Autodesk Inventor part; units mm, degrees
ref_plane "YZ Plane" through (0, 0, 0) normal (1, 0, 0) x (0, 1, 0)
ref_plane "XZ Plane" through (0, 0, 0) normal (0, 1, 0) x (-1, 0, 0)
ref_plane "XY Plane" through (0, 0, 0) normal (0, 0, 1) x (1, 0, 0)
sketch "Szkic1" plane through (0, 0, 0) normal (0, 0, 1) x (1, 0, 0)
  line L0 (0, 0) -> (-30, 30)
  line L1 (-30, 30) -> (-30, 27.1716)
  line L2 (-30, 27.1716) -> (-2.8284, 0)
  line L3 (-2.8284, 0) -> (0, 0)
  line L4 (-30, 27.1716) -> (-30.8284, 28)
  line L5 (-30.8284, 28) -> (-30.8284, 30)
  line L6 (-30.8284, 30) -> (-30, 30)
  dimension "d0" = 2
  dimension "d1" = 30
  dimension "d2" = 45
  dimension "d3" = 2
extrude "Wyciągnięcie proste1" add sketch "Szkic1" along normal blind 180.257
sketch "Szkic2" plane through (-30.8284, 28, 0) normal (-1, 0, 0) x (0, 0, 1)
  line L0 (0, 0) -> (0, -28)
  line L1 (0, 2) -> (180.257, 2)
  line L2 (0, -28) -> (0, 2)
  line L3 (0, 2) -> (30, 2)
  line L4 (0, 0) -> (180.257, 0)
  line L5 (30, 2) -> (0, -28)
  line L6 (180.257, 2) -> (180.257, -20)
  line L7 (180.257, 0) -> (180.257, -28)
  line L8 (180.257, 2) -> (142.1519, 2)
  line L9 (180.257, -20) -> (142.1519, 2)
  dimension "d6" = 45
  dimension "d7" = 30
  dimension "d8" = 22
extrude "Wyciągnięcie proste2" cut sketch "Szkic2" against normal through all contours L4 L5 L0 | L2 L1 L5 L4 | L9 L1 L6 L4 | L4 L6 L9
sketch "Szkic3" plane through (0, 0, 0) normal (0.7071, 0.7071, 0) x (-0.7071, 0.7071, 0)
  line L0 (42.4264, 30) -> (42.4264, 142.1519) construction
  line L1 (42.4264, 115.152) -> (23.012, 115.152) construction
  circle A0 centre (32.012, 135.152) radius 1.6
  circle A1 centre (23.012, 115.152) radius 1.6
  circle A2 centre (32.012, 33.9815) radius 1.6
  line L2 (41.598, 28) -> (41.598, 145.616)
  point P0 (0, 0)
  dimension "d17" = 3.2
  dimension "d37" = 9.586
  dimension "d38" = 5.9815
  dimension "d39" = 10.464
  dimension "d40" = 30.464
  dimension "d41" = 18.586
extrude "Wyciągnięcie proste3" cut sketch "Szkic3" against normal through all
chamfer "Faza1" distance 1.85 distance2 1.75 1 edges at (-15.1406, 15.1406, 115.152) measured on face at (-5.0469, 5.0469, 98.4697)
chamfer "Faza2" distance 1.85 distance2 1.75 1 edges at (-21.5045, 21.5045, 135.152) measured on face at (-4.6108, 4.6108, 98.4697)
chamfer "Faza3" distance 1.85 distance2 1.75 1 edges at (-21.5045, 21.5045, 33.9815) measured on face at (-4.6108, 4.6108, 98.4697)
sketch "Szkic4" plane through (-30.8284, 28, 28) normal (-1, 0, 0) x (0, 0, 1)
  circle A0 centre (34.7574, -13) radius 19.25
  line L0 (-28, -28) -> (152.257, -28)
  dimension "d29" = 62.7574
  dimension "d30" = 38.5
  dimension "d31" = 15
extrude "Wyciągnięcie proste4" cut sketch "Szkic4" against normal blind 22.5
sketch "Szkic5" plane through (0, 0, 0) normal (0.7071, 0.7071, 0) x (-0.7071, 0.7071, 0)
  line L0 (9.7782, 79.4999) -> (9.7782, 46.0149)
  line L1 (9.7782, 79.4999) -> (9.7782, 46.0149)
  ellipse E0 centre (16.4957, 62.7574) end of major axis (16.4957, 43.5074) minor radius 13.6118 (9.7782, 46.0149) -> (11.7782, 44.7005) ccw
  ellipse E1 centre (16.4957, 62.7574) end of major axis (16.4957, 43.5074) minor radius 13.6118 (11.7782, 80.8143) -> (9.7782, 79.4999) ccw
  ellipse E2 centre (23.2132, 62.7574) end of major axis (50.4368, 62.7574) minor radius 19.25 (41.598, 76.9547) -> (9.7782, 79.4999) ccw
  ellipse E3 centre (32.4056, 62.7574) end of major axis (32.4056, 43.5074) minor radius 13.6118 (43.0122, 74.8223) -> (41.598, 76.9547) ccw
  ellipse E4 centre (32.4056, 62.7574) end of major axis (32.4056, 43.5074) minor radius 13.6118 (41.598, 48.5601) -> (43.0122, 50.6925) ccw
  line L2 (43.0122, 74.8223) -> (43.0122, 50.6925)
  ellipse E5 centre (23.2132, 62.7574) end of major axis (50.4368, 62.7574) minor radius 19.25 (9.7782, 46.0149) -> (41.598, 48.5601) ccw
  ellipse E6 centre (21.2132, 62.7574) end of major axis (48.4368, 62.7574) minor radius 19.25 (11.7782, 44.7005) -> (42.4264, 50.6925) ccw
  ellipse E7 centre (21.2132, 62.7574) end of major axis (48.4368, 62.7574) minor radius 19.25 (42.4264, 74.8223) -> (11.7782, 80.8143) ccw
  line L3 (42.4264, 30) -> (42.4264, 50.6925)
  line L4 (42.4264, 74.8223) -> (42.4264, 50.6925)
  point P0 (0, 0)
  point P1 (41.598, 48.5601)
extrude "Wyciągnięcie proste5" cut sketch "Szkic5" against normal through all
properties part number "Bok2mm"
Here's how the part is built. I have some questions about the finished solid (model axes, mm). Round coordinates to 2 decimals unless told otherwise and drop trailing zeros. Loops run counter-clockwise (first coordinate to the right, second up) from the corner with the lowest first, then second, coordinate; pieces in that order, holes last. Notation, with made-up numbers: (23, -21.75) -> (32, -21.75) arc R7 ccw to (32, -15.75) -> close; hole circle Ø8 at (-14, -28). An arc over 180 degrees is marked (long way). Write each question's results on one line, items separated by ' | '.
(1) If I drill on L1, parallel to X at y = 2.5, z = 98.5; L2, parallel to X at y = 11, z = 87; L3, parallel to Y at x = -6.5, z = 128.5, over which ranges is the centre line in solid material (lowest first)?
Worked answers:
L1: -5.33 to -2.5 | L2: -13.83 to -11 | L3: 3.67 to 6.5
(2) We'd pull the mould along Z, two halves only. Please class faces 1 (the face through (-19.467, 18.134, 162.705)), 2 (the face through (-13.91, 11.08, 88.87)), 3 (the face through (-23.5, 21.2, 32.3)): released by +Z, released by -Z, zero draft, split by the parting line, or undercut.
Worked answers:
face 1: released by +Z | face 2: zero draft | face 3: undercut
(3) If we section it at B-B, the plane z = 17: List the corners of the cut face in (x, y) for me.
Worked answers:
outline: (-19.83, 17) -> (-2.83, 0) -> (0, 0) -> (-17, 17) -> close
(4) If we section it at A-A, the plane z = 107.5: List the corners of the cut face in (x, y) for me, then the cut area to 3 significant figures.
Worked answers:
outline: (-30.83, 28) -> (-2.83, 0) -> (0, 0) -> (-30, 30) -> (-30.83, 30) -> close | area: 82.9 mm2
(5) If we section it at C-C, the plane z = 166: List the corners of the cut face in (x, y) for me.
Worked answers:
outline: (-19.06, 16.23) -> (-2.83, 0) -> (0, 0) -> (-16.23, 16.23) -> close
(6) For P1, Ø8, axis at x = -15.5, y = 3, coming from the +Z side; P2, Ø10, axis at y = 23.5, z = 90, coming from the +X side; P3, Ø3, axis at y = 15, z = 110, coming from the +X side; P4, Ø4, axis at x = -15.5, z = 117.5, coming from the +Y side, each with a flat end and sliding along its axis, tell me the tip position at first contact or that it passes through.
Worked answers:
P1: through | P2: x = -18.5 | P3: x = -13.5 | P4: y = 17.36
